Verification items for this drawing (mm, ordinates from the low corner). A direction names the side the tool comes from. Give positions to 0.01 mm unless a question says otherwise; leave off trailing zeros. Write each loop counter-clockwise with the first axis right and the second up, starting at its lowest first coordinate (ties: lowest second). Pieces come first, ordered by that corner, then holes. Notation, with made-up numbers: (59.5, 68) -> (97.5, 68) arc R3 cw to (97.5, 73) -> close; hole circle Ø9 at (10, 17). An arc over 180 degrees is marked (long way). Answer as a JSON object with one key per item and string values.
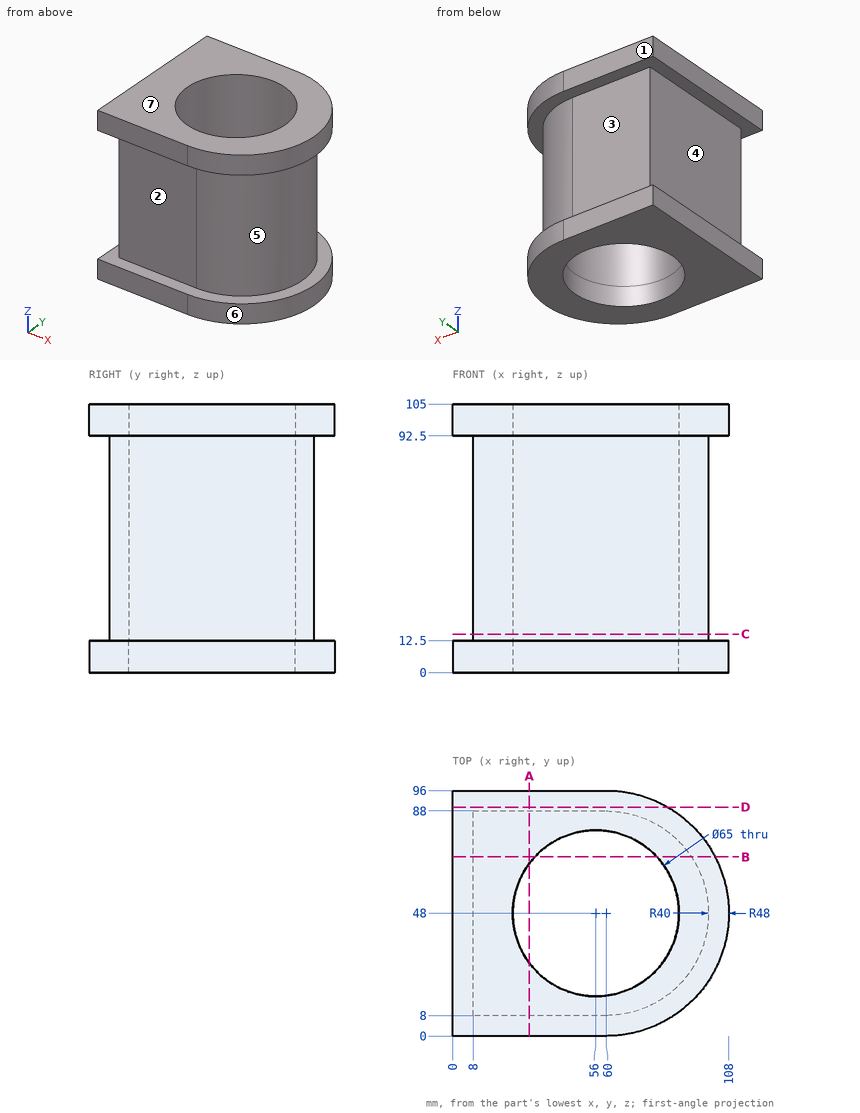
1. Sectioned sample at B-B, the plane y = 70. Enter the section's corners in (x, z), plus the area to 3 significant figures.
Determined:
{"outline": "(0, 0) -> (32.08, 0) -> (32.08, 105) -> (0, 105) -> (0, 92.5) -> (8, 92.5) -> (8, 12.5) -> (0, 12.5) -> close; (79.92, 0) -> (102.66, 0) -> (102.66, 12.5) -> (93.41, 12.5) -> (93.41, 92.5) -> (102.66, 92.5) -> (102.66, 105) -> (79.92, 105) -> close", "area": "4,380 mm^2"}
2. Scan lines: L1, parallel to Y at x = 56, z = 44; L2, parallel to Y at x = 56, z = 8.5; L3, parallel to X at y = 36.5, z = 48. Record each from-to range of solid material in increasing order. Write a range as [from, to].
Determined:
{"L1": "[8, 15.5], [80.5, 88]", "L2": "[0, 15.5], [80.5, 96]", "L3": "[8, 25.6], [86.4, 98.31]"}
3. Go/stop test with flat-tipped pins: P1, Ø10, axis at x = 32, z = 30.5, coming from the -Y side; P2, Ø10, axis at x = 88.5, z = 83.5, coming from the -Y side; P3, Ø1.5, axis at x = 45, z = 34, coming from the +Y side. Record where each tip stops, or that it passes through.
Determined:
{"P1": "y = 8", "P2": "y = 15.63", "P3": "y = 88"}
4. Sectioned sample at D-D, the plane y = 89.5. Enter the section's corners in (x, z), plus the area to 3 significant figures.
Determined:
{"outline": "(0, 0) -> (84.12, 0) -> (84.12, 12.5) -> (0, 12.5) -> close; (0, 92.5) -> (84.12, 92.5) -> (84.12, 105) -> (0, 105) -> close", "area": "2,100 mm^2"}
5. Access from +Z, -Z, +X, -X, +Y, -Y to the whole of each face (thin tool, end or side, straight path). Record for the marked faces 1, 2 and 3.
Determined:
{"face 1": "+Z, -Z, +X, -X, +Y", "face 2": "+X, -X, -Y", "face 3": "+X, -X, +Y"}
6. Sectioned sample at A-A, the plane x = 30. Enter the section's corners in (y, z).
Determined:
{"outline": "(0, 0) -> (28.5, 0) -> (28.5, 105) -> (0, 105) -> (0, 92.5) -> (8, 92.5) -> (8, 12.5) -> (0, 12.5) -> close; (67.5, 0) -> (96, 0) -> (96, 12.5) -> (88, 12.5) -> (88, 92.5) -> (96, 92.5) -> (96, 105) -> (67.5, 105) -> close"}
7. Sectioned sample at C-C, the plane z = 15. Enter the section's corners in (x, y), plus the area to 3 significant figures.
Determined:
{"outline": "(8, 8) -> (60, 8) arc R40 ccw to (60, 88) -> (8, 88) -> close; hole circle Ø65 at (56, 48)", "area": "3,350 mm^2"}
8. Mould release check, pull along Z, two halves, no side actions. Record for the marked faces 4, 5, 6 and 7: released by +Z, released by -Z, zero draft, split by the parting line, or undercut.
Determined:
{"face 4": "undercut", "face 5": "undercut", "face 6": "zero draft", "face 7": "released by +Z"}
